Verification items for the finished model (mm, model axes). Face numbers are marked on the shaded views. A direction names the side the tool comes from. Coordinates: 2 decimals unless noted, no trailing zeros. Loops run counter-clockwise (first coordinate to the right, second up) from the corner with the lowest first, then second, coordinate; pieces in that order, holes last. Notation, with made-up numbers: M 38,11.25 L 61,11.25 A14 ccw 61,30.25 Z; hole C -35,-9 d3. An arc over 180 degrees is marked long. Write item = value, one per line. Start each with the question number.
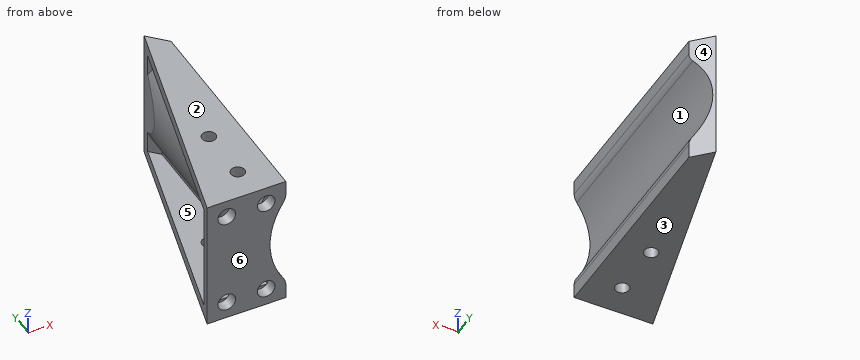
Autodesk Inventor part; units mm, degrees
ref_plane "Work Plane1" through (0, 0, -17) normal (0, 0, 1) x (1, 0, 0)
ref_plane "YZ Plane" through (0, 0, 0) normal (1, 0, 0) x (0, 1, 0)
ref_plane "XZ Plane" through (0, 0, 0) normal (0, 1, 0) x (-1, 0, 0)
sketch "Sketch1" plane through (0, 0, 0) normal (0, 1, 0) x (-1, 0, 0)
  line L0 (0, 0) -> (-20, 0)
  line L1 (-20, 0) -> (-20, -34)
  line L2 (-20, -34) -> (0, -34)
  line L3 (0, -34) -> (0, 0)
  dimension "d0" = 34
  dimension "d1" = 20
extrude "Extrusion1" add sketch "Sketch1" along normal blind 60
chamfer "Chamfer1" distance 4.5 angle 45 1 edges at (20, 60, -17)
sketch "Sketch3" plane through (0, 0, 0) normal (0, 0, 1) x (1, 0, 0)
  line L0 (0, 60) -> (15.5, 60)
  line L1 (15.5, 60) -> (0, 0)
  line L2 (0, 0) -> (20, 0)
  line L3 (20, 0) -> (0, 0)
  line L4 (0, 0) -> (0, 60)
  line L5 (0, 60) -> (20, 60)
  line L6 (20, 60) -> (20, 0)
extrude "Extrusion2" cut sketch "Sketch3" against normal blind 60 contours L0 L1 L4
sketch "Sketch8" plane through (0, 0, 0) normal (0, -1, 0) x (1, 0, 0)
  line L0 (20, 0) -> (20, -34)
  line L1 (20, -17) -> (36, -17) construction
  circle A0 centre (36, -17) radius 20
  point P0 (0, 0)
  point P1 (20, -29)
  point P2 (20, -5)
  dimension "d44" = 40
  dimension "d45" = 16
extrude "Extrusion7" cut sketch "Sketch8" against normal through all contours L0 A0 picked at (19.2708, -19.7731)
shell "Shell2" thickness 3 removed faces 1 at (10.3333, 40, -22.6667)
sketch "Sketch9" plane through (0, 0, 0) normal (0, -1, 0) x (1, 0, 0)
  circle A0 centre (5, -4.5) radius 2.25
  line L0 (0, 0) -> (20, 0)
  line L1 (0, -34) -> (0, 0)
  line L2 (5, -4.5) -> (15, -4.5) construction
  line L3 (14.629, -8.4982) -> (14.629, -3)
  line L4 (5, -4.5) -> (15, -4.5) construction
  circle A1 centre (15, -4.5) radius 2.25
  line L5 (0, -17) -> (10, -17) construction
  circle A2 centre (5, -29.5) radius 2.25
  circle A3 centre (15, -29.5) radius 2.25
  dimension "d49" = 4.5
  dimension "d50" = 4.5
  dimension "d51" = 5
  dimension "d52" = 10
  dimension "d53" = 360
  dimension "d54" = 4.5
  dimension "d56" = 25
extrude "Extrusion8" cut sketch "Sketch9" against normal blind 3
fillet "Fillet2" radius 4 2 edges at (20, 27.75, -5) (20, 27.75, -29)
sketch "Sketch10" plane through (20, 0, 0) normal (0, 0, 1) x (1, 0, 0)
  circle A0 centre (-8, 8) radius 1.75
  line L0 (-8, 8) -> (-8, 22) construction
  circle A1 centre (-8, 22) radius 1.75
  point P0 (-20, 0)
  dimension "d60" = 3.5
  dimension "d61" = 12
  dimension "d62" = 8
  dimension "d64" = 3.5
extrude "Extrusion9" cut sketch "Sketch10" against normal blind 3
ref_plane "Work Plane1" through (0, 0, -17) normal (0, 0, 1) x (1, 0, 0)
mirror "Mirror1" about plane through (0, 0, -17) normal (0, 0, 1) of "Extrusion9"
properties part number "Gripper"
Q1. Sectioned sample at C-C on x = 5.5. Record the cut outline in (y, z).
Q2. Gauge pin test, flat ends, axial feed: pin 1 (1 mm diameter, centred on x = 3.5, z = -28, fed in from +Y); pin 2 (1.1 mm diameter, centred on y = 39.5, z = -3.5, fed in from -X) (3 decimals); pin 3 (0.5 mm diameter, centred on x = 16, z = -29.5, fed in from -Y). Record the tip position at first contact, or that the pin passes through.
Q3. Sectioned sample at B-B on x = 12. Record the cut outline in (y, z).
Q4. Mould release check, pull along Z, two halves, no side actions. Record for the marked faces 1, 2, 3 and 4: +Z half, -Z half, draft (parallel to the pull), parting line (faces both ways), or undercut.
Q5. Sectioned sample at D-D on z = -17.5. Record the cut outline in (x, y) (3 decimals), plus the area to 3 significant figures.
Q6. Sectioned sample at A-A on y = 22. Record the cut outline in (x, z).
Q7. Scan lines: L1, parallel to Z at x = 15, y = 1.45; L2, parallel to Z at x = 12.5, y = 16; L3, parallel to X at y = 0.75, z = -4.5. Record each from-to range of solid material in increasing order. Write a range as [from, to].
Q8. Set-up check for the marked faces 5 and 6: record each of +Z, -Z, +X, -X, +Y, -Y from which the full face is reachable in a straight line by a thin tool's end or side.
Solutions:
q1.outline = M 0,-34 L 21.29,-34 L 21.29,-31 L 3,-31 L 3,-31.69 L 0,-31.69 Z; M 0,-27.31 L 3,-27.31 L 3,-6.69 L 0,-6.69 Z; M 0,-2.31 L 3,-2.31 L 3,-3 L 21.29,-3 L 21.29,0 L 0,0 Z
q2.pin_1 = 3
q2.pin_2 = 10.145
q2.pin_3 = 55.01
q3.outline = M 0,-34 L 6.25,-34 L 6.25,-31 L 3,-31 L 3,-3 L 6.25,-3 L 6.25,0 L 0,0 Z; M 9.75,-34 L 20.25,-34 L 20.25,-31 L 9.75,-31 Z; M 9.75,-3 L 20.25,-3 L 20.25,0 L 9.75,0 Z; M 23.75,-34 L 46.45,-34 L 46.45,-31 L 23.75,-31 Z; M 23.75,-3 L 46.45,-3 L 46.45,0 L 23.75,0 Z
q4.face_1 = undercut
q4.face_2 = +Z half
q4.face_3 = -Z half
q4.face_4 = draft
q5.outline = M 0,0 L 16.006,0 L 16.006,59.494 L 15.5,60 L 13.005,50.344 L 13.005,3 L 0.775,3 Z
q5.area = 206 mm²
q6.outline = M 5.68,-34 L 10.25,-34 L 10.25,-31 L 5.68,-31 Z; M 5.68,-3 L 10.25,-3 L 10.25,0 L 5.68,0 Z; M 13.75,-34 L 20,-34 L 20,-30.27 A4 ccw 19.33,-28.06 A20 cw 19.33,-5.94 A4 ccw 20,-3.73 L 20,0 L 13.75,0 L 13.75,-3 L 17,-3 L 17,-4.04 A23 ccw 17,-29.96 L 17,-31 L 13.75,-31 Z
q7.L1 = [-34, -31.75], [-27.25, -6.75], [-2.25, 0]
q7.L2 = [-34, -31], [-3, 0]
q7.L3 = [0.19, 2.75], [7.25, 12.75], [17.25, 19.93]
q8.face_5 = -X
q8.face_6 = +Z, -Z, +X, -X, -Y
